Geometry: final body of the model. Coordinates: model frame, mm. Face numbers are marked on the shaded views. A direction names the side the tool comes from. Coordinates: 2 decimals unless noted, no trailing zeros. Write each loop counter-clockwise with the first axis right and the second up, starting at its lowest first coordinate (ties: lowest second). Pieces come first, ordered by that corner, then holes. Notation, with made-up numbers: (76, 73) - (103, 73) arc R26 cw to (103, 109) - close; hole circle Ø5 at (46.25, 68.25). An arc over 180 degrees is marked (long way). Answer as a JSON object with one key per item and string values. Group by question number.
Item 1: Section A-A on y = -3.75. Return loops of the section in (x, z).
Item 2: Mould query, pull axis X, two halves, no side actions, for the marked faces 1, 2, 3 and 4. Classes: pulls with the +X half, pulls with the -X half, needs draft (parallel to the pull), parting line crosses it, or undercut.
Item 3: Section B-B on z = 5. Return loops of the section in (x, y), and give its area (3 significant figures).
Item 4: Section C-C on y = 0.25. Return loops of the section in (x, z), and give its area (3 significant figures).
Item 5: Set-up query: the marked faces 5, 6 and 7. Return all of +Z, -Z, +X, -X, +Y, -Y with unobstructed straight access to the full face (end or side cutting, diameter ignored); none if empty.
Item 6: Section D-D on x = 13.4. Return loops of the section in (y, z), and give its area (3 significant figures).
Item 7: First-contact query: pin 1 Ø4 at (y, z) = (-0.5, 5) entering from -X; pin 2 Ø4 at (x, z) = (-13.4, 5) entering from +Y; pin 3 Ø5 at (y, z) = (3.5, 6.5) entering from +X; pin 4 Ø3 at (x, z) = (1.5, 3) entering from -Y. Flat tips, straight axial feed; report the tip coordinate or a pass-through.
Item 8: Line query: line 1 along X through (y, z) = (-4.3, 5); line 2 along X through (y, z) = (2.5, 4.25); line 3 along X through (y, z) = (-3.5, 0.5). Output: solid intervals per line, ascending. Write a range as from..to.
```python
from build123d import *

# Parameters (mm, degrees)
BOSS_EXTRUDE1_DEPTH = 10
SKETCH2_R           = 1.65
CUT_EXTRUDE1_DEPTH  = 3


with BuildPart() as part:
    # Sketch1 → Boss-Extrude1 (new body)
    with BuildSketch(Plane.XY):
        Polygon((17.5, -5.15), (6.3, -5.15), (6.3, 5.15), (-6.3, 5.15), (-6.3, -5.15), (-17.5, -5.15), (-17.5, -2.15), (-9.3, -2.15), (-9.3, 8.15), (9.3, 8.15), (9.3, -2.15), (17.5, -2.15), align=None)
    extrude(amount=BOSS_EXTRUDE1_DEPTH)

    # Sketch2 → Cut-Extrude1 (cut)
    with BuildSketch(Plane(origin=(0, -2.15, 0), x_dir=(1, 0, 0), z_dir=(0, 1, 0))):
        with Locations(Location((13.4, -5, 0), (0, 0, 270))):
            Circle(SKETCH2_R)
        with Locations(Location((-13.4, -5, 0), (0, 0, 270))):
            Circle(SKETCH2_R)
    extrude(amount=-CUT_EXTRUDE1_DEPTH, mode=Mode.SUBTRACT)


solid = part.part
```
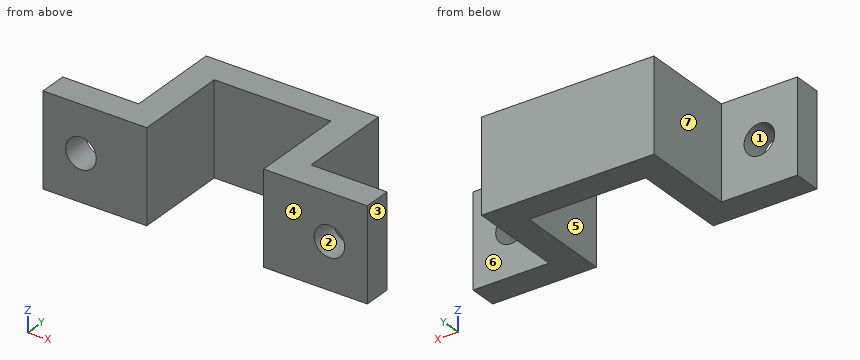
Checks:
{
 "1": {"outline": "(-17.5, 0) - (-6.3, 0) - (-6.3, 10) - (-17.5, 10) - close; (6.3, 0) - (17.5, 0) - (17.5, 10) - (6.3, 10) - close; hole circle Ø3.3 at (-13.4, 5); hole circle Ø3.3 at (13.4, 5)"},
 "2": {"face 1": "undercut", "face 2": "undercut", "face 3": "pulls with the +X half", "face 4": "needs draft"},
 "3": {"outline": "(-17.5, -5.15) - (-15.05, -5.15) - (-15.05, -2.15) - (-17.5, -2.15) - close; (-11.75, -5.15) - (-6.3, -5.15) - (-6.3, 5.15) - (6.3, 5.15) - (6.3, -5.15) - (11.75, -5.15) - (11.75, -2.15) - (9.3, -2.15) - (9.3, 8.15) - (-9.3, 8.15) - (-9.3, -2.15) - (-11.75, -2.15) - close; (15.05, -5.15) - (17.5, -5.15) - (17.5, -2.15) - (15.05, -2.15) - close", "area": "147 mm^2"},
 "4": {"outline": "(-9.3, 0) - (-6.3, 0) - (-6.3, 10) - (-9.3, 10) - close; (6.3, 0) - (9.3, 0) - (9.3, 10) - (6.3, 10) - close", "area": "60.0 mm^2"},
 "5": {"face 5": "+Z, -Z, -Y", "face 6": "+Z, -Z, +X, +Y", "face 7": "+Z, -Z, -X, +Y"},
 "6": {"outline": "(-5.15, 0) - (-2.15, 0) - (-2.15, 3.35) - (-5.15, 3.35) - close; (-5.15, 6.65) - (-2.15, 6.65) - (-2.15, 10) - (-5.15, 10) - close", "area": "20.1 mm^2"},
 "7": {"pin 1": "x = -17.5", "pin 2": "y = -2.15", "pin 3": "x = 9.3", "pin 4": "y = 5.15"},
 "8": {"line 1": "-17.5..-15.05, -11.75..-6.3, 6.3..11.75, 15.05..17.5", "line 2": "-9.3..-6.3, 6.3..9.3", "line 3": "-17.5..-6.3, 6.3..17.5"}
}
